Read the model definition and answer for the solid it produces. Units are mm, in the model's axes. Face numbers are marked on the shaded views. A direction names the side the tool comes from. Coordinates: 2 decimals unless noted, no trailing zeros. Order: outer loops, then holes, each group sorted by start corner. A loop starts at its lowest first (then second) coordinate and runs counter-clockwise, first axis right, second up. Notation, with made-up numbers: (-26.75, 71.5) -> (30.25, 71.5) arc R14 cw to (30.25, 93.5) -> close; hole circle Ø10 at (12, 7). An arc over 180 degrees is marked (long way). Use CSV: the item, a comma, the result in double quotes.
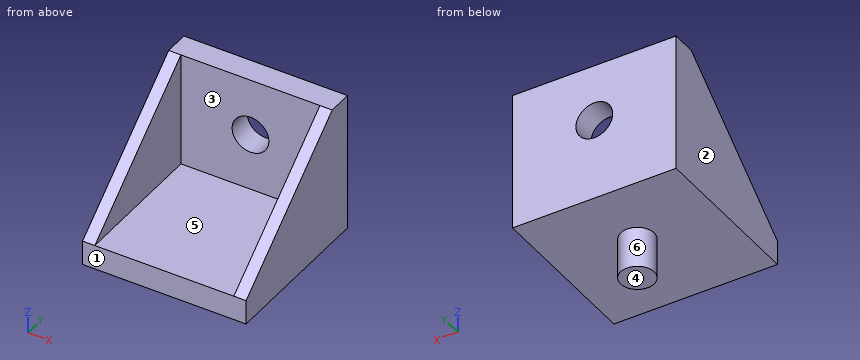
```python
from build123d import *

# Parameters (mm, degrees)
SKETCH_1_W          = 20
SKETCH_1_H          = 20
EXTRUDE_1_DEPTH     = 17
CUT_EXTRUDE_1_DEPTH = 20
SKETCH_3_W          = 17
SKETCH_3_H          = 17
CUT_EXTRUDE_2_DEPTH = 14
HOLE_WIZARD_M4_1_D  = 4.5
SKETCH_9_R          = 2.05
EXTRUDE_3_DEPTH     = 5


with BuildPart() as part:
    # 스케치1 → 보스-돌출1 (new body)
    with BuildSketch(Plane.XY):
        Rectangle(SKETCH_1_W, SKETCH_1_H)
    extrude(amount=EXTRUDE_1_DEPTH)

    # 스케치2 → 컷-돌출1 (cut)
    with BuildSketch(Plane(origin=(10, 0, 0), x_dir=(0, 0, -1), z_dir=(1, 0, 0))):
        Polygon((-17, 7), (-3, -10), (-17, -10), align=None)
    extrude(amount=-CUT_EXTRUDE_1_DEPTH, mode=Mode.SUBTRACT)

    # 스케치3 → 컷-돌출2 (cut)
    with BuildSketch(Plane.XY.offset(17)):
        with Locations((0, -1.5)):
            Rectangle(SKETCH_3_W, SKETCH_3_H)
    extrude(amount=-CUT_EXTRUDE_2_DEPTH, mode=Mode.SUBTRACT)

    # M4 여유 구멍1 (through all)
    with Locations(Plane(origin=(0, 7, 0), x_dir=(-1, 0, 0), z_dir=(0, -1, 0))):
        with Locations((0, -10)):
            Hole(HOLE_WIZARD_M4_1_D / 2)

    # 스케치9 → 보스-돌출3 (add)
    with BuildSketch(Plane(origin=(0, 0, 0), x_dir=(-1, 0, 0), z_dir=(0, 0, -1))):
        with Locations((0, 1.5)):
            Circle(SKETCH_9_R)
    extrude(amount=EXTRUDE_3_DEPTH)


solid = part.part
```
Item 1: Find section A-A, the plane x = 0. Give the vertices of the cut face in (y, z), then the cut area to 3 significant figures.
Return value:
outline,"(-10, 0) -> (-0.55, 0) -> (-0.55, -5) -> (3.55, -5) -> (3.55, 0) -> (10, 0) -> (10, 7.75) -> (7, 7.75) -> (7, 3) -> (-10, 3) -> close; (7, 12.25) -> (10, 12.25) -> (10, 17) -> (7, 17) -> close"
area,"109 mm^2"
Item 2: Find section D-D, the plane x = -7.25. Give the vertices of the cut face in (y, z).
Return value:
outline,"(-10, 0) -> (10, 0) -> (10, 17) -> (7, 17) -> (7, 3) -> (-10, 3) -> close"
Item 3: A tool of negligible diameter and unlimited length cuts with its end or side. For the marked faces 4, 5 and 6, from which of +Z, -Z, +X, -X, +Y, -Y can it reach the whole face along a straight path? Write none if from no direction.
Return value:
face 4,"-Z, +X, -X, +Y, -Y"
face 5,"+Z, -Y"
face 6,"-Z"
Item 4: Find section B-B, the plane z = 10. Give the vertices of the cut face in (x, y).
Return value:
outline,"(-10, -1.5) -> (-8.5, -1.5) -> (-8.5, 7) -> (-2.25, 7) -> (-2.25, 10) -> (-10, 10) -> close; (2.25, 7) -> (8.5, 7) -> (8.5, -1.5) -> (10, -1.5) -> (10, 10) -> (2.25, 10) -> close"
Item 5: Straight lines are drawn through the part: line 1 along X through (y, z) = (1.5, 11.5); line 2 along X through (y, z) = (7.8, 10); line 3 along Z through (x, y) = (0, 8.35). For each, find the intervals that lie inside material, in ascending order.
Return value:
line 1,"x = -10 to -8.5, 8.5 to 10"
line 2,"x = -10 to -2.25, 2.25 to 10"
line 3,"z = 0 to 7.75, 12.25 to 17"
Item 6: Each of these flat-tipped pins is pushed along its axis until it touches: P1, Ø4, axis at x = 5.5, y = -4, coming from the +Z side; P2, Ø5, axis at x = 0.5, z = 10, coming from the -Y side; P3, Ø12, axis at x = -0.5, z = 5.5, coming from the -Y side. Where does it stop, or does it pass through?
Return value:
P1,"stops at z = 3"
P2,"stops at y = 7"
P3,"stops at y = -10"
Item 7: Find section C-C, the plane z = 15.75. Give the vertices of the cut face in (x, y).
Return value:
outline,"(-10, 5.48) -> (-8.5, 5.48) -> (-8.5, 7) -> (8.5, 7) -> (8.5, 5.48) -> (10, 5.48) -> (10, 10) -> (-10, 10) -> close"
Item 8: The mould has two halves that part along X. Classify the marked faces 1, 2 and 3: +X half, -X half, draft (parallel to the pull), parting line (faces both ways), or undercut.
Return value:
face 1,"draft"
face 2,"-X half"
face 3,"undercut"
